Could you check a few things on this model? Use its own coordinates, in mm. Face numbers are marked on the shaded views. A direction names the side the tool comes from. Coordinates: 2 decimals unless noted, no trailing zeros. Loops run counter-clockwise (first coordinate to the right, second up) from the corner with the lowest first, then second, coordinate; pieces in that order, holes last. Notation, with made-up numbers: (71, 84.5) -> (91, 84.5) arc R23 ccw to (91, 103.5) -> close; hole circle Ø6 at (64.25, 7.5). An arc over 180 degrees is marked (long way). One line per question, with ' | ' between items. Start each with the question number.
(1) Suppose I cut it at D-D (y = 123). Please give me the cut outline in (x, z) (3 decimals).
(2) I'm going to push flat-ended pins straight in: pin 1 Ø11.5 at (x, z) = (6.5, 2.5) entering from +Y; pin 2 Ø1.5 at (x, z) = (-5.5, 7) entering from -Y; pin 3 Ø2 at (x, z) = (-12, 9.5) entering from +Y; pin 4 Ø5 at (x, y) = (-6.5, 74) entering from +Z. Where does each tip first touch, or does it pass through?
(3) If I drill on line 1 along Y through (x, z) = (2, -11); line 2 along Z through (x, y) = (1, 84); line 3 along Z through (x, y) = (-13, 36.5), over which ranges is the centre line in solid material (lowest first)?
(4) If we mould it in two halves opening along Z, with no side actions, what happens to the marked faces 3 and 4? For each: pulls with the +Z half, pulls with the -Z half, needs draft (parallel to the pull), parting line crosses it, or undercut.
(5) Suppose I cut it at A-A (x = 0). Please give me the cut outline in (y, z) (3 decimals).
(6) Suppose I cut it at C-C (z = 0). Please give me the cut outline in (x, y).
(7) Which directions (+Z, -Z, +X, -X, +Y, -Y) give clear straight access to the entire face, cutting with the end or side of a thin tool? Please do the marked faces 1 and 2.
(8) Suppose I cut it at B-B (y = 92). Please give me the cut outline in (x, z).
```python
from build123d import *

# Parameters (mm, degrees)
SKETCH1_R           = 19
BOSS_EXTRUDE1_DEPTH = 100
SKETCH2_R           = 6
BOSS_EXTRUDE2_DEPTH = 7
SKETCH3_R           = 3
BOSS_EXTRUDE3_DEPTH = 27
CUT_EXTRUDE1_DEPTH  = 22


with BuildPart() as part:
    # Sketch1 → Boss-Extrude1 (new body)
    with BuildSketch(Plane(origin=(0, 0, 0), x_dir=(1, 0, 0), z_dir=(0, 1, 0))):
        Circle(SKETCH1_R)
    extrude(amount=BOSS_EXTRUDE1_DEPTH)

    # Sketch2 → Boss-Extrude2 (add)
    with BuildSketch(Plane(origin=(0, 100, 0), x_dir=(1, 0, 0), z_dir=(0, 1, 0))):
        with Locations((0, -9.825)):
            Circle(SKETCH2_R)
    extrude(amount=BOSS_EXTRUDE2_DEPTH)

    # Sketch3 → Boss-Extrude3 (add)
    with BuildSketch(Plane(origin=(0, 107, 0), x_dir=(1, 0, 0), z_dir=(0, 1, 0))):
        with Locations((0, -9.825)):
            Circle(SKETCH3_R)
    extrude(amount=BOSS_EXTRUDE3_DEPTH)

    # Sketch4 → Cut-Extrude1 (cut)
    with BuildSketch(Plane(origin=(0, 134, 0), x_dir=(1, 0, 0), z_dir=(0, 1, 0))):
        Polygon((-9.150633985, -13.135072473), (10.849366015, -10.314966588), (10.988990103, -11.30517117), (-9.011009897, -14.125277054), align=None)
    extrude(amount=-CUT_EXTRUDE1_DEPTH, mode=Mode.SUBTRACT)


solid = part.part
```
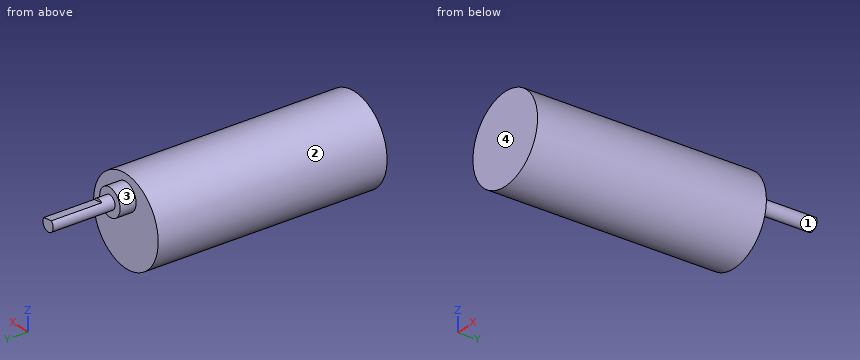
Checks:
1) outline: (-1.935, 12.118) arc R3 ccw (long way) to (2.493, 11.493) -> close
2) pin 1: stops at y = 107 | pin 2: stops at y = 0 | pin 3: stops at y = 100 | pin 4: stops at z = 18.57
3) line 1: y = 0 to 100 | line 2: z = -18.97 to 18.97 | line 3: z = -13.86 to 13.86
4) face 3: parting line crosses it | face 4: needs draft
5) outline: (0, -19) -> (100, -19) -> (100, 3.825) -> (107, 3.825) -> (107, 6.825) -> (134, 6.825) -> (134, 11.845) -> (112, 11.845) -> (112, 12.825) -> (107, 12.825) -> (107, 15.825) -> (100, 15.825) -> (100, 19) -> (0, 19) -> close
6) outline: (-19, 0) -> (19, 0) -> (19, 100) -> (-19, 100) -> close
7) face 1: +Y | face 2: +Y, -Y
8) outline: circle Ø38 at (0, 0)
